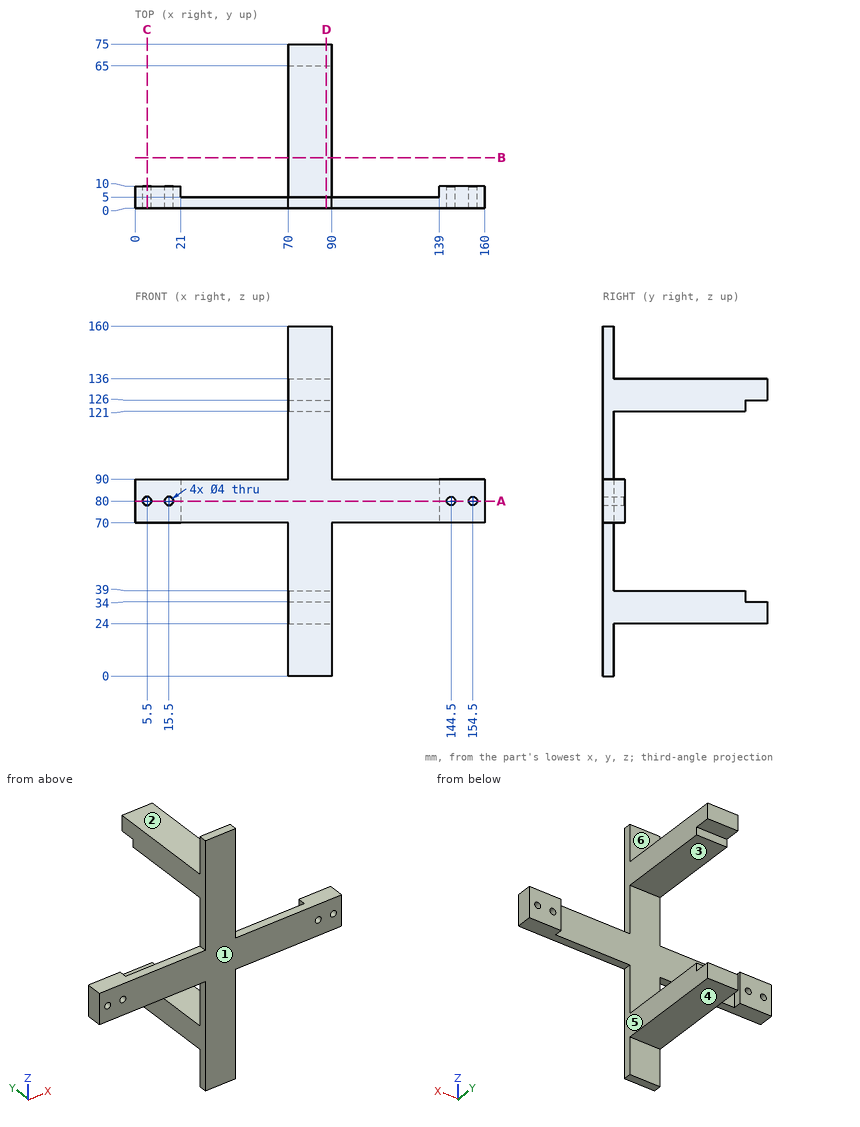
Geometry check sheet. Reference: drawing and pictorial views, mm from the part's lowest x, y, z. A direction names the side the tool comes from. Give positions to 0.01 mm unless a question says otherwise; leave off trailing zeros. Write each loop counter-clockwise with the first axis right and the second up, starting at its lowest first coordinate (ties: lowest second). Pieces come first, ordered by that corner, then holes. Notation, with made-up numbers: (81, 17.5) -> (140, 17.5) arc R17 ccw to (140, 39.5) -> close; hole circle Ø5 at (-21, 66.5). An arc over 180 degrees is marked (long way). One line per question, with ' | ' between items.
Item 1: Sectioned sample at A-A, the plane z = 80. Record the boundary of the cut face in (x, y).
Determined:
outline: (0, 0) -> (3.5, 0) -> (3.5, 10) -> (0, 10) -> close; (7.5, 0) -> (13.5, 0) -> (13.5, 10) -> (7.5, 10) -> close; (17.5, 0) -> (142.5, 0) -> (142.5, 10) -> (139, 10) -> (139, 5) -> (21, 5) -> (21, 10) -> (17.5, 10) -> close; (146.5, 0) -> (152.5, 0) -> (152.5, 10) -> (146.5, 10) -> close; (156.5, 0) -> (160, 0) -> (160, 10) -> (156.5, 10) -> close
Item 2: Sectioned sample at C-C, the plane x = 5.5. Record the boundary of the cut face in (y, z), plus the area to 3 significant figures.
Determined:
outline: (0, 70) -> (10, 70) -> (10, 78) -> (0, 78) -> close; (0, 82) -> (10, 82) -> (10, 90) -> (0, 90) -> close | area: 160 mm^2
Item 3: Scan lines: line 1 along X through (y, z) = (6, 80); line 2 along Z through (x, y) = (154.5, 3.25); line 3 along X through (y, z) = (50, 123.5). Record each from-to range of solid material in increasing order.
Determined:
line 1: 0 to 3.5, 7.5 to 13.5, 17.5 to 21, 139 to 142.5, 146.5 to 152.5, 156.5 to 160 | line 2: 70 to 78, 82 to 90 | line 3: 70 to 90
Item 4: Draft check along Z on the marked faces 1, 2 and 3. Enter one of: released by +Z, released by -Z, zero draft, split by the parting line, or undercut.
Determined:
face 1: zero draft | face 2: released by +Z | face 3: undercut
Item 5: Access from +Z, -Z, +X, -X, +Y, -Y to the whole of each face (thin tool, end or side, straight path). Record for the marked faces 4, 5 and 6.
Determined:
face 4: -Z, +X, -X, +Y | face 5: -Z, +X, +Y, -Y | face 6: +Z, +X, -X, +Y
Item 6: Sectioned sample at B-B, the plane y = 23. Record the boundary of the cut face in (x, z).
Determined:
outline: (70, 24) -> (90, 24) -> (90, 39) -> (70, 39) -> close; (70, 121) -> (90, 121) -> (90, 136) -> (70, 136) -> close
Item 7: Depth check by flat-ended pin: pin 1 (5 mm diameter, centred on x = 22, y = 4, fed in from +Z); pin 2 (22 mm diameter, centred on x = 84.5, z = 12, fed in from +Y); pin 3 (10 mm diameter, centred on y = 12, z = 121, fed in from +X). Enter the tip coordinate at first touch or a pass-through.
Determined:
pin 1: z = 90 | pin 2: y = 5 | pin 3: x = 90
Item 8: Sectioned sample at D-D, the plane x = 87.5. Record the boundary of the cut face in (y, z), plus the area to 3 significant figures.
Determined:
outline: (0, 0) -> (5, 0) -> (5, 24) -> (75, 24) -> (75, 34) -> (65, 34) -> (65, 39) -> (5, 39) -> (5, 121) -> (65, 121) -> (65, 126) -> (75, 126) -> (75, 136) -> (5, 136) -> (5, 160) -> (0, 160) -> close | area: 2,800 mm^2
